For this review, take the finished solid that the model builds, in its own axes (mm). A direction names the side the tool comes from. Give positions to 0.01 mm unless a question says otherwise; leave off trailing zeros. Loops run counter-clockwise (first coordinate to the right, second up) from the corner with the lowest first, then second, coordinate; pieces in that order, holes last. Notation, with made-up numbers: M 2.5,6 L 55.5,6 A25 cw 55.5,19 Z; hole C 56,75 d5. An arc over 180 degrees is marked long. Use CSV: the item, a comma, the result in double quotes. Start each with the question number.
1. Take a section at A-A, the plane y = 24. Write out the cut boundary in (x, z), and give its area (3 significant figures).
2. Take a section at C-C, the plane z = 6. Write out the cut boundary in (x, y).
3. Insertion check: P1, Ø8, axis at x = -9, z = 28, coming from the -Y side; P2, Ø5, axis at x = -10.5, z = 25.5, coming from the +Y side; P3, Ø2, axis at x = 5, y = 9.5, coming from the -Z side; P4, Ø1.8, axis at x = 10, y = 46.14, coming from the -Z side. Each pin has a flat end and moves straight along its axis. Give the tip position at first contact, or say it passes through.
4. The part is to be moulded in two halves that separate along X. For faces 5 (the face through (-20.907, 19.701, 36.165)), 6 (the face through (0, 38.64, 4)), 7 (the face through (20.907, 19.701, 36.165)), 8 (the face through (-13, 31, 0)), say which applies: pulls with the +X half, pulls with the -X half, needs draft (parallel to the pull), parting line crosses it, or undercut.
5. Take a section at D-D, the plane y = 4.5. Write out the cut boundary in (x, z), and give its area (3 significant figures).
6. To check wall thickness, follow line 1 (Y direction, x = 0, z = 4); line 2 (Z direction, x = -13, y = 46). State the ranges of each line that lie inside material, in increasing order. Write a range as [from, to].
7. Tool access review of faces 1 (the face through (-11.11, 47.15, 3.76)), 2 (the face through (0.267, 61.138, 3.944)), 3 (the face through (14.98, 27.38, 45.84)), 4 (the face through (0, 50, 8)): name each direction out of +Z, -Z, +X, -X, +Y, -Y from which nothing blocks a thin tool from reaching the whole face with its end or side.
8. Take a section at B-B, the plane x = 0. Write out the cut boundary in (y, z).
from build123d import *

# Parameters (mm, degrees)
F0_R      = 1.5
F0_R_2    = 2.5
F1_DEPTH  = 8
F2_W      = 55
F2_H      = 8
F3_DEPTH  = 8
F4_R      = 4.75
F4_R_2    = 1.5
F5_DEPTH  = 8
F8_REACH  = 140.1940387091
F11_REACH = 140.1940387091
F13_DEPTH = 25


with BuildPart() as f1:
    # F0 (on Top) → F1 (new body)
    with BuildSketch(Plane.XY):
        Polygon((-27.5, 8), (-27.5, 0), (27.5, 0), (27.5, 8), (19.1259515677, 8), (-19.1259515677, 8), align=None)
        with BuildLine():
            Line((-16.4747191004, 43.64), (-27.5, 8))
            Line((-27.5, 8), (-19.1259515677, 8))
            Line((-19.1259515677, 8), (-9.6474272477, 38.64))
            Line((-9.6474272477, 38.64), (9.6474272477, 38.64))
            Line((9.6474272477, 38.64), (19.1259515677, 8))
            Line((19.1259515677, 8), (27.5, 8))
            Line((27.5, 8), (16.4747191004, 43.64))
            Line((16.4747191004, 43.64), (14.3299863823, 50.5730001446))
            ThreePointArc((14.3299863823, 50.5730001446), (0, 61.14), (-14.3299863823, 50.5730001446))
            Line((-14.3299863823, 50.5730001446), (-16.4747191004, 43.64))
        make_face()
        with Locations((-10, 46.14)):
            Circle(F0_R, mode=Mode.SUBTRACT)
        with Locations((0, 46.14)):
            Circle(F0_R_2, mode=Mode.SUBTRACT)
        with Locations((10, 46.14)):
            Circle(F0_R, mode=Mode.SUBTRACT)
    extrude(amount=F1_DEPTH)

    # F2 (on face) → F3 (join)
    with BuildSketch(Plane.XZ):
        with BuildLine():
            Line((27.5, 8), (19.8895027624, 80.0994475138))
            ThreePointArc((19.8895027624, 80.0994475138), (0, 98), (-19.8895027624, 80.0994475138))
            Line((-19.8895027624, 80.0994475138), (-27.5, 8))
            Line((-27.5, 8), (27.5, 8))
        make_face()
        with Locations((0, 4)):
            Rectangle(F2_W, F2_H)
    extrude(amount=-F3_DEPTH)

    # F4 (on face) → F5 (cut, through all)
    with BuildSketch(Plane.XZ):
        with Locations((0, 78)):
            Circle(F4_R)
        with Locations((-5.6568542495, 83.6568542495)):
            Circle(F4_R_2)
        with Locations((6.7175144213, 84.7175144213)):
            Circle(F4_R_2)
        with Locations((5.6568542495, 72.3431457505)):
            Circle(F4_R_2)
        with Locations((-6.7175144213, 71.2824855787)):
            Circle(F4_R_2)
    extrude(amount=-F5_DEPTH, mode=Mode.SUBTRACT)

    f8_end = Plane(origin=(14.3866894077, 23.32, 4), x_dir=(0.295533343, -0.9553324255, 0), z_dir=(-0.9553324255, -0.295533343, 0))
    # F7 (on 3pt) → F8 (join, up to a plane its end follows)
    with BuildSketch(Plane(origin=(27.8443578743, 8.6136887495, 2.9391266645), x_dir=(-0.2924175497, 0.9557924714, -0.0308662969), z_dir=(0.95051185, 0.2940420916, 0.1003318064))):
        Polygon((-0.6420732198, 77.5690607735), (-0.6420732198, 5.0690607735), (43.900022914, 6.4515483908), align=None)
    f8_long = extrude(amount=-F8_REACH, mode=Mode.PRIVATE)
    add(split(f8_long, bisect_by=f8_end, keep=Keep.BOTTOM, mode=Mode.PRIVATE))

    f11_end = Plane(origin=(-14.3866894077, 23.32, 4), x_dir=(0.295533343, 0.9553324255, 0), z_dir=(0.9553324255, -0.295533343, 0))
    # F10 (on 3pt) → F11 (join, up to a plane its end follows)
    with BuildSketch(Plane(origin=(-27.8443578743, 8.6136887495, 2.9391266645), x_dir=(0.2924175497, 0.9557924714, -0.0308662969), z_dir=(0.95051185, -0.2940420916, -0.1003318064))):
        Polygon((-0.6420732198, 77.5690607735), (-0.6420732198, 5.0690607735), (43.900022914, 6.4515483908), align=None)
    f11_long = extrude(amount=F11_REACH, mode=Mode.PRIVATE)
    add(split(f11_long, bisect_by=f11_end, keep=Keep.BOTTOM, mode=Mode.PRIVATE))

    # F12 (on face) → F13 (cut)
    with BuildSketch(Plane.XY.offset(8)):
        with BuildLine():
            Line((-18.02147568, 38.64), (-9.6474272477, 38.64))
            Line((-9.6474272477, 38.64), (9.6474272477, 38.64))
            Line((9.6474272477, 38.64), (18.02147568, 38.64))
            Line((18.02147568, 38.64), (14.3299863823, 50.5730001446))
            ThreePointArc((14.3299863823, 50.5730001446), (0, 61.14), (-14.3299863823, 50.5730001446))
            Line((-14.3299863823, 50.5730001446), (-18.02147568, 38.64))
        make_face()
    extrude(amount=F13_DEPTH, mode=Mode.SUBTRACT)


solid = f1.part
Result set:
1,outline,"M -22.55,0 L -14.18,0 L -14.18,50.81 L -17.8,53 L -22.55,8 Z; M 14.18,0 L 22.55,0 L 22.55,8 L 17.8,53 L 14.18,50.81 Z"
1,area,"666 mm2"
2,outline,"M -27.5,0 L 27.5,0 L 27.5,8 L 14.33,50.57 A15 ccw -14.33,50.57 L -27.5,8 Z; hole M -19.13,8 L 19.13,8 L 9.65,38.64 L -9.65,38.64 Z; hole C -10,46.14 d3; hole C 0,46.14 d5; hole C 10,46.14 d3"
3,P1,"y = 0"
3,P2,"y = 38.64"
3,P3,"through"
3,P4,"z = 7.36"
4,face 5,"pulls with the -X half"
4,face 6,"undercut"
4,face 7,"pulls with the +X half"
4,face 8,"needs draft"
5,outline,"M -27.5,0 L 27.5,0 L 27.5,8 L 19.89,80.1 A20 ccw -19.89,80.1 L -27.5,8 Z; hole C -6.72,71.28 d3; hole C -5.66,83.66 d3; hole C 0,78 d9.5; hole C 5.66,72.34 d3; hole C 6.72,84.72 d3"
5,area,"4,300 mm2"
6,line 1,"[0, 8], [38.64, 43.64], [48.64, 61.14]"
6,line 2,"[0, 8]"
7,face 1,"-Z"
7,face 2,"+Z, -Z, +Y"
7,face 3,"+Z, +Y"
7,face 4,"+Z, +X, -X, +Y"
8,outline,"M 0,0 L 8,0 L 8,73.25 L 0,73.25 Z; M 0,82.75 L 8,82.75 L 8,98 L 0,98 Z; M 38.64,0 L 43.64,0 L 43.64,8 L 38.64,8 Z; M 48.64,0 L 61.14,0 L 61.14,8 L 48.64,8 Z"
